Verification items for the finished model (mm, model axes). A direction names the side the tool comes from. Give positions to 0.01 mm unless a question says otherwise; leave off trailing zeros. Write each loop counter-clockwise with the first axis right and the second up, starting at its lowest first coordinate (ties: lowest second). Pieces come first, ordered by that corner, then holes. Notation, with made-up numbers: (49.25, 66) - (63.25, 66) arc R13 ccw to (63.25, 85) - close; hole circle Ø7 at (85, -5). An arc over 180 degrees is marked (long way). Put each result on its own line as item: value.
from build123d import *

# Parameters (mm, degrees)
SKETCH1_W           = 20
SKETCH1_H           = 20
SKETCH1_W_2         = 17
SKETCH1_H_2         = 17
BOSS_EXTRUDE2_DEPTH = 2
SKETCH1_4_W         = 20
SKETCH1_4_H         = 20
SKETCH1_4_W_2       = 17
SKETCH1_4_H_2       = 17
BOSS_EXTRUDE3_DEPTH = 10
SKETCH2_W           = 12
SKETCH2_H           = 1.5
CUT_EXTRUDE1_DEPTH  = 8


with BuildPart() as part:
    # Sketch1 → Boss-Extrude2 (new body)
    # profile 1 of 2: a face of its own
    with BuildSketch(Plane(origin=(0, 0, 0), x_dir=(1, 0, 0), z_dir=(0, 1, 0))):
        with Locations((8.5, 8.5)):
            Rectangle(SKETCH1_W, SKETCH1_H)
        with Locations((8.5, 8.5)):
            Rectangle(SKETCH1_W_2, SKETCH1_H_2, mode=Mode.SUBTRACT)
    # profile 2 of 2: a face of its own
    with BuildSketch(Plane(origin=(0, 0, 0), x_dir=(1, 0, 0), z_dir=(0, 1, 0))):
        with Locations((8.5, 8.5)):
            Rectangle(SKETCH1_W_2, SKETCH1_H_2)
    extrude(amount=BOSS_EXTRUDE2_DEPTH)

    # Sketch1<4> → Boss-Extrude3 (add)
    with BuildSketch(Plane(origin=(0, 0, 0), x_dir=(1, 0, 0), z_dir=(0, 1, 0))):
        with Locations((8.5, 8.5)):
            Rectangle(SKETCH1_4_W, SKETCH1_4_H)
        with Locations((8.5, 8.5)):
            Rectangle(SKETCH1_4_W_2, SKETCH1_4_H_2, mode=Mode.SUBTRACT)
    extrude(amount=BOSS_EXTRUDE3_DEPTH)

    # Sketch2 → Cut-Extrude1 (cut)
    with BuildSketch(Plane(origin=(0, 10, 0), x_dir=(1, 0, 0), z_dir=(0, 1, 0))):
        with Locations((8.577582313, 17.75)):
            Rectangle(SKETCH2_W, SKETCH2_H)
        with Locations((8.44538549, -0.75)):
            Rectangle(SKETCH2_W, SKETCH2_H)
    extrude(amount=-CUT_EXTRUDE1_DEPTH, mode=Mode.SUBTRACT)


solid = part.part
Q1. Go/stop test with flat-tipped pins: pin 1 Ø5 at (x, z) = (10.5, -4.5) entering from +Y; pin 2 Ø6 at (x, z) = (10, -12.5) entering from -Y. Record where each tip stops, or that it passes through.
Answers follow:
pin 1: stops at y = 2
pin 2: stops at y = 0
Q2. Set-up check for faces 4 (the face through (14.445, 6, 1)), 5 (the face through (16, 6, -17)), 6 (the face through (2.445, 6, 1)): record each of +Z, -Z, +X, -X, +Y, -Y from which the full face is reachable in a straight line by a thin tool's end or side.
Answers follow:
face 4: +Z, -Z, +Y
face 5: +Y
face 6: +Z, +Y
Q3. Section check A-A, the plane y = 3.5. Record the cut outline in (x, z).
Answers follow:
outline: (-1.5, -18.5) - (2.58, -18.5) - (2.58, -17) - (0, -17) - (0, 0) - (2.45, 0) - (2.45, 1.5) - (-1.5, 1.5) - close; (14.45, 0) - (17, 0) - (17, -17) - (14.58, -17) - (14.58, -18.5) - (18.5, -18.5) - (18.5, 1.5) - (14.45, 1.5) - close
Q4. Scan lines: line 1 along X through (y, z) = (3, -14); line 2 along Z through (x, y) = (0.25, 6.5); line 3 along Y through (x, z) = (7, -2). Record each from-to range of solid material in increasing order.
Answers follow:
line 1: x = -1.5 to 0, 17 to 18.5
line 2: z = -18.5 to -17, 0 to 1.5
line 3: y = 0 to 2
Q5. Release check for a two-part mould opening along X. For faces 1 (the face through (-0.4, 10, -8.6)), 2 (the face through (14.578, 6, -18)), 3 (the face through (18.5, 5, -8)) record: released by +X, released by -X, zero draft, split by the parting line, or undercut.
Answers follow:
face 1: zero draft
face 2: undercut
face 3: released by +X
Q6. Section check C-C, the plane x = 15.5. Record the cut outline in (y, z), plus the area to 3 significant figures.
Answers follow:
outline: (0, -18.5) - (10, -18.5) - (10, -17) - (2, -17) - (2, 0) - (10, 0) - (10, 1.5) - (0, 1.5) - close
area: 64.0 mm2
Q7. Section check B-B, the plane z = -8.75. Record the cut outline in (x, y).
Answers follow:
outline: (-1.5, 0) - (18.5, 0) - (18.5, 10) - (17, 10) - (17, 2) - (0, 2) - (0, 10) - (-1.5, 10) - close
